from build123d import *

# Parameters (mm, degrees)
F1_DEPTH = 400


with BuildPart() as f1:
    # F0 (on Front) → F1 (new body)
    with BuildSketch(Plane.XZ):
        with BuildLine():
            Line((-103.557974, -56.594891), (-140.819733, -56.594891))
            ThreePointArc((-140.819733, -56.594891), (-140.834136, -56.594905), (-140.848538, -56.594891))
            ThreePointArc((-140.848538, -56.594891), (-146.318086, -54.211179), (-148.31709, -48.589611))
            Line((-148.31709, -48.589611), (-148.31709, -40.039665))
            ThreePointArc((-148.31709, -40.039665), (-146.120392, -34.736367), (-140.817094, -32.539669))
            Line((-140.817094, -32.539669), (-136.722556, -32.539669))
            Line((-136.722556, -32.539669), (-136.722556, -29.539669))
            Line((-136.722556, -29.539669), (-140.817094, -29.539669))
            ThreePointArc((-140.817094, -29.539669), (-148.241712, -32.615047), (-151.31709, -40.039665))
            Line((-151.31709, -40.039665), (-151.31709, -48.496935))
            ThreePointArc((-151.31709, -48.496935), (-151.324869, -48.653976), (-151.330295, -48.811115))
            ThreePointArc((-151.330295, -48.811115), (-153.747489, -54.327682), (-159.327372, -56.594891))
            Line((-159.327372, -56.594891), (-209.665096, -56.594891))
            Line((-209.665096, -56.594891), (-209.665096, -60.594891))
            Line((-209.665096, -60.594891), (-9.665096, -60.594891))
            Line((-9.665096, -60.594891), (190.334904, -60.594891))
            Line((190.334904, -60.594891), (190.334904, -56.594891))
            Line((190.334904, -56.594891), (139.997181, -56.594891))
            ThreePointArc((139.997181, -56.594891), (134.417297, -54.327682), (132.000103, -48.811115))
            ThreePointArc((132.000103, -48.811115), (131.994677, -48.653976), (131.986898, -48.496935))
            Line((131.986898, -48.496935), (131.986898, -40.039665))
            ThreePointArc((131.986898, -40.039665), (128.911521, -32.615047), (121.486903, -29.539669))
            Line((121.486903, -29.539669), (117.392364, -29.539669))
            Line((117.392364, -29.539669), (117.392364, -32.539669))
            Line((117.392364, -32.539669), (121.486903, -32.539669))
            ThreePointArc((121.486903, -32.539669), (126.7902, -34.736367), (128.986898, -40.039665))
            Line((128.986898, -40.039665), (128.986898, -48.589611))
            ThreePointArc((128.986898, -48.589611), (126.987895, -54.211179), (121.518346, -56.594891))
            ThreePointArc((121.518346, -56.594891), (121.503944, -56.594905), (121.489541, -56.594891))
            Line((121.489541, -56.594891), (84.227782, -56.594891))
            Line((84.227782, -56.594891), (31.486903, -56.594891))
            Line((31.486903, -56.594891), (-9.665096, -56.594891))
            Line((-9.665096, -56.594891), (-50.817094, -56.594891))
            Line((-50.817094, -56.594891), (-59.151821, -56.594891))
            Line((-59.151821, -56.594891), (-103.557974, -56.594891))
        make_face()
    extrude(amount=F1_DEPTH)


solid = f1.part
Can you work these out from the model? Positions are in its coordinate system, mm. A direction names the side the tool comes from. Give positions to 0.01 mm unless a question says otherwise; leave off trailing zeros. Loops run counter-clockwise (first coordinate to the right, second up) from the corner with the lowest first, then second, coordinate; pieces in that order, holes last. Notation, with made-up numbers: (0.25, 26.5) - (38.25, 26.5) arc R12 cw to (38.25, 38.5) - close; hole circle Ø9 at (-17.5, 73.5). An arc over 180 degrees is marked (long way). Return JSON: item names as keys, results as strings.
1. We'd pull the mould along Z, two halves only. Please class faces 1 (the face through (-184, -197, -56.595)), 2 (the face through (-148.317, -197, -44)), 3 (the face through (-11, 0, -58)): +Z half, -Z half, draft (parallel to the pull), parting line (faces both ways), or undercut.
Output values:
{"face 1": "+Z half", "face 2": "undercut", "face 3": "draft"}
2. I'm going to push flat-ended pins straight in: pin 1 Ø25 at (x, y) = (177.5, -191.5) entering from +Z; pin 2 Ø2 at (y, z) = (-323.5, -49) entering from +X; pin 3 Ø2.5 at (y, z) = (-129.5, -31) entering from +X. Where does each tip first touch, or does it pass through?
Output values:
{"pin 1": "stops at z = -56.59", "pin 2": "stops at x = 132.12", "pin 3": "stops at x = 128.53"}
3. I want a section at B-B on x = -8.5. Please give me the cut outline in (y, z), and give its area (3 significant figures).
Output values:
{"outline": "(-400, -60.59) - (0, -60.59) - (0, -56.59) - (-400, -56.59) - close", "area": "1,600 mm²"}
4. If I drill on line 1 (Z direction, x = -141, y = -44); line 2 (X direction, y = -285, z = -46.5); line 3 (Z direction, x = -188, y = -240), over which ranges is the centre line in solid material (lowest first)?
Output values:
{"line 1": "z = -60.59 to -56.59, -32.54 to -29.54", "line 2": "x = -151.32 to -148.32, 128.99 to 131.99", "line 3": "z = -60.59 to -56.59"}
5. For faces 4 (the face through (166, -197, -56.595)), 5 (the face through (128.987, -197, -44)), 6 (the face through (-11, -400, -58)), which set-ups out of +Z, -Z, +X, -X, +Y, -Y let a thin tool reach every point of the face, with its end or its side?
Output values:
{"face 4": "+Z, +X, +Y, -Y", "face 5": "+Y, -Y", "face 6": "+Z, -Z, +X, -X, -Y"}
